```python
from build123d import *

# Parameters (mm, degrees)
SKETCH2_W                      = 60
SKETCH2_H                      = 32
BOSS_EXTRUDE1_DEPTH            = 10
CBORE_FOR_M3_SHCS1_D           = 3.4
CBORE_FOR_M3_SHCS1_CBORE_D     = 6.5
CBORE_FOR_M3_SHCS1_CBORE_DEPTH = 5
SKETCH6_W                      = 17
SKETCH6_H                      = 12
CUT_EXTRUDE2_DEPTH             = 2
CUT_EXTRUDE4_DEPTH             = 5
M5_CLEARANCE_HOLE1_D           = 5.5
SKETCH12_R                     = 2
BOSS_EXTRUDE2_DEPTH            = 2.5
M2X0_4_TAPPED_HOLE1_D          = 1.6
BOSS_EXTRUDE3_DEPTH            = 5
BOSS_EXTRUDE4_DEPTH            = 6.5
FILLET1_R                      = 4
M2X0_4_TAPPED_HOLE2_D          = 1.6
M2X0_4_TAPPED_HOLE2_DEPTH      = 5.2
M2X0_4_TAPPED_HOLE2_TIP        = 0.480688495
CUT_EXTRUDE5_DEPTH             = 3
CHAMFER1_SIZE                  = 1
BOSS_EXTRUDE5_DEPTH            = 10
SKETCH26_R                     = 5.5
CUT_EXTRUDE7_DEPTH             = 14
SKETCH27_R                     = 4
CUT_EXTRUDE8_DEPTH             = 14
FILLET2_R                      = 3
SKETCH28_W                     = 6
SKETCH28_H                     = 6
BOSS_EXTRUDE6_DEPTH            = 10
CUT_EXTRUDE9_DEPTH             = 52.000867623
CUT_EXTRUDE10_REACH            = 76.738
SKETCH30_R                     = 1.6
SKETCH31_R                     = 1.4
CUT_EXTRUDE11_DEPTH            = 5


with BuildPart() as part:
    # Sketch2 → Boss-Extrude1 (new body)
    with BuildSketch(Plane(origin=(0, 0, 0), x_dir=(1, 0, 0), z_dir=(0, 1, 0))):
        Rectangle(SKETCH2_W, SKETCH2_H)
    extrude(amount=BOSS_EXTRUDE1_DEPTH)

    # CBORE for M3 SHCS1 (through all)
    with Locations(Plane(origin=(0, 0, 0), x_dir=(-1, 0, 0), z_dir=(0, -1, 0))):
        with Locations((12.5, 12.5), (12.5, -12.5), (-12.5, -12.5), (-12.5, 12.5)):
            CounterBoreHole(CBORE_FOR_M3_SHCS1_D / 2, CBORE_FOR_M3_SHCS1_CBORE_D / 2, CBORE_FOR_M3_SHCS1_CBORE_DEPTH)

    # Sketch6 → Cut-Extrude2 (cut)
    with BuildSketch(Plane(origin=(0, 0, 0), x_dir=(-1, 0, 0), z_dir=(0, -1, 0))):
        with Locations((0, 10)):
            Rectangle(SKETCH6_W, SKETCH6_H)
    extrude(amount=-CUT_EXTRUDE2_DEPTH, mode=Mode.SUBTRACT)

    # Sketch8 → Cut-Extrude4 (cut)
    with BuildSketch(Plane(origin=(0, 0, -16), x_dir=(-1, 0, 0), z_dir=(0, 0, -1))):
        Polygon((17.265727793, 5), (19.632863896, 0.9), (24.367136104, 0.9), (26.734272207, 5), (24.367136104, 9.1), (19.632863896, 9.1), align=None)
        Polygon((-17.265727793, 5), (-19.632863896, 9.1), (-24.367136104, 9.1), (-26.734272207, 5), (-24.367136104, 0.9), (-19.632863896, 0.9), align=None)
    extrude(amount=-CUT_EXTRUDE4_DEPTH, mode=Mode.SUBTRACT)

    # M5 Clearance Hole1 (through all)
    with Locations(Plane(origin=(0, 0, -11), x_dir=(-1, 0, 0), z_dir=(0, 0, -1))):
        with Locations((22, 5), (-22, 5)):
            Hole(M5_CLEARANCE_HOLE1_D / 2)

    # Sketch12 → Boss-Extrude2 (add)
    with BuildSketch(Plane.XZ):
        with Locations(Location((10.5, -6.5, 0), (0, 0, 180))):
            Circle(SKETCH12_R)
        with Locations((-10.5, -6.5)):
            Circle(SKETCH12_R)
        with Locations(Location((10.5, 6, 0), (0, 0, 90))):
            Circle(SKETCH12_R)
        with Locations(Location((-10.5, 6, 0), (0, 0, 90))):
            Circle(SKETCH12_R)
    extrude(amount=BOSS_EXTRUDE2_DEPTH)

    # M2x0.4 Tapped Hole1 (through all)
    with Locations(Plane(origin=(0, -2.5, 0), x_dir=(-1, 0, 0), z_dir=(0, -1, 0))):
        with Locations((-10.5, -6), (-10.5, 6.5), (10.5, -6), (10.5, 6.5)):
            Hole(M2X0_4_TAPPED_HOLE1_D / 2)

    # Sketch15 → Boss-Extrude3 (add)
    with BuildSketch(Plane(origin=(0, 0, -16), x_dir=(-1, 0, 0), z_dir=(0, 0, -1))):
        Polygon((-13.5, 0), (-13.5, 10), (13.5, 10), (13.5, 0), (8.5, 0), (8.5, 2), (-8.5, 2), (-8.5, 0), align=None)
    extrude(amount=BOSS_EXTRUDE3_DEPTH)

    # Sketch19 → Boss-Extrude4 (add)
    with BuildSketch(Plane(origin=(0, 0, -21), x_dir=(-1, 0, 0), z_dir=(0, 0, -1))):
        Polygon((13.5, 0), (13.5, -6.7), (8.5, -6.7), (8.5, 0), (8.5, 10), (13.5, 10), align=None)
        Polygon((-8.5, 0), (-8.5, 10), (-13.5, 10), (-13.5, 0), (-13.5, -6.7), (-8.5, -6.7), align=None)
    extrude(amount=BOSS_EXTRUDE4_DEPTH)

    # Fillet1
    fillet1_edges = [part.edges().sort_by_distance(p)[0] for p in [
        (-11, 0, -21),
        (11, 0, -21),
    ]]
    fillet(fillet1_edges, radius=FILLET1_R)

    # M2x0.4 Tapped Hole2
    with Locations(Plane(origin=(0, 0, -27.5), x_dir=(-1, 0, 0), z_dir=(0, 0, -1))):
        with Locations((10.75, -4.7), (-10.75, -4.7), (-10.75, 8), (10.75, 8)):
            Hole(M2X0_4_TAPPED_HOLE2_D / 2, depth=M2X0_4_TAPPED_HOLE2_DEPTH)
            with Locations((0, 0, -(M2X0_4_TAPPED_HOLE2_DEPTH + M2X0_4_TAPPED_HOLE2_TIP / 2))):  # 118° drill point
                Cone(0, M2X0_4_TAPPED_HOLE2_D / 2, M2X0_4_TAPPED_HOLE2_TIP, mode=Mode.SUBTRACT)

    # Sketch23 → Cut-Extrude5 (cut)
    with BuildSketch(Plane(origin=(0, 0, -27.5), x_dir=(-1, 0, 0), z_dir=(0, 0, -1))):
        Polygon((8.5, 8), (11.5, 5), (11.5, -1.7), (8.5, -4.7), (-8.5, -4.7), (-11.5, -1.7), (-11.5, 5), (-8.5, 8), align=None)
    extrude(amount=-CUT_EXTRUDE5_DEPTH, mode=Mode.SUBTRACT)

    # Chamfer1
    # the kernel refuses this chamfer: 1 mm, written as the material it adds along each edge
    with BuildSketch(Plane(origin=(10.5, 0, 6), x_dir=(0, 0, 1), z_dir=(1, 0, 0))) as chamfer1_piece_1:
        Polygon((2 + CHAMFER1_SIZE, 0), (2, CHAMFER1_SIZE), (2, 0), align=None)
    revolve(axis=Axis((10.5, 0, 6), (0, -1, 0)))
    with BuildSketch(Plane(origin=(-10.5, 0, -6.5), x_dir=(1, 0, 0), z_dir=(0, 0, -1))) as chamfer1_piece_2_section:
        Polygon((2 + CHAMFER1_SIZE, 0), (2, CHAMFER1_SIZE), (2, 0), align=None)
    chamfer1_piece_2 = revolve(axis=Axis((-10.5, 0, -6.5), (0, -1, 0)), mode=Mode.PRIVATE)
    chamfer1_piece_2 = split(chamfer1_piece_2, bisect_by=Plane(origin=(-8.5, -0.487052851, -6.5), z_dir=(-1, 0, 0)), keep=Keep.TOP, mode=Mode.PRIVATE)
    add(chamfer1_piece_2)
    with BuildSketch(Plane(origin=(-10.5, 0, 6), x_dir=(0, 0, 1), z_dir=(1, 0, 0))) as chamfer1_piece_3:
        Polygon((2 + CHAMFER1_SIZE, 0), (2, CHAMFER1_SIZE), (2, 0), align=None)
    revolve(axis=Axis((-10.5, 0, 6), (0, -1, 0)))
    with BuildSketch(Plane(origin=(10.5, 0, -6.5), x_dir=(-1, 0, 0), z_dir=(0, 0, 1))) as chamfer1_piece_4_section:
        Polygon((2 + CHAMFER1_SIZE, 0), (2, CHAMFER1_SIZE), (2, 0), align=None)
    chamfer1_piece_4 = revolve(axis=Axis((10.5, 0, -6.5), (0, -1, 0)), mode=Mode.PRIVATE)
    chamfer1_piece_4 = split(chamfer1_piece_4, bisect_by=Plane(origin=(8.5, -0.487052851, -6.5), z_dir=(1, 0, 0)), keep=Keep.TOP, mode=Mode.PRIVATE)
    add(chamfer1_piece_4)

    # Sketch25 → Boss-Extrude5 (add)
    with BuildSketch(Plane.XZ):
        Polygon((-30, 0.5), (-30, -6.5), (-30, -13.5), (-41.771263836, -13.5), (-41.771263836, 0.5), align=None)
    extrude(amount=-BOSS_EXTRUDE5_DEPTH)

    # Sketch26 → Cut-Extrude7 (cut)
    with BuildSketch(Plane(origin=(-34.168169597, -5.889190106, 16), x_dir=(-0.888296712324418, -0.45927001956760705, 0), z_dir=(0.45927001956760705, -0.888296712324418, 0))):
        with Locations(Location((-5.5, 22.5, 0), (0, 0, 180))):
            Circle(SKETCH26_R)
    extrude(amount=-CUT_EXTRUDE7_DEPTH, mode=Mode.SUBTRACT)

    # Sketch27 → Cut-Extrude8 (cut, along a direction that is not the sketch's normal)
    with BuildSketch(Plane(origin=(-11.234235046, 21.728686027, 0), x_dir=(0.888296712324418, 0.45927001956760705, 0), z_dir=(0.45927001956760705, -0.888296712324418, 0))):
        with Locations((-27.556201174, -6.5)):
            Circle(SKETCH27_R)
    extrude(amount=-CUT_EXTRUDE8_DEPTH, dir=(0, -1, 0), mode=Mode.SUBTRACT)

    # Fillet2
    fillet2_edges = [part.edges().sort_by_distance(p)[0] for p in [
        (-13.5, 5, -16),
        (13.5, 5, -16),
        (-41.771263836, 5, 0.5),
        (-41.771263836, 5, -13.5),
    ]]
    fillet(fillet2_edges, radius=FILLET2_R)

    # Sketch28 → Boss-Extrude6 (add)
    with BuildSketch(Plane.XZ):
        with Locations((-35.771263836, 3.5)):
            Rectangle(SKETCH28_W, SKETCH28_H)
    extrude(amount=-BOSS_EXTRUDE6_DEPTH)

    # Sketch29 → Cut-Extrude9 (cut, through all)
    with BuildSketch(Plane.XZ):
        Polygon((-30, 0.5), (-31.125452896, -5.882760545), (-33.813152902, -5.408846518), (-32.771263836, 0.5), align=None)
    extrude(amount=-CUT_EXTRUDE9_DEPTH, mode=Mode.SUBTRACT)

    # Sketch30 → Cut-Extrude10 (cut, up to next)
    with BuildSketch(Plane.ZY.offset(38.771263836), mode=Mode.PRIVATE) as cut_extrude10_sk1:
        with Locations((3.5, 5)):
            Circle(SKETCH30_R)
    cut_extrude10_tool1 = extrude(cut_extrude10_sk1.sketch, amount=-CUT_EXTRUDE10_REACH, mode=Mode.PRIVATE) & part.part
    add(cut_extrude10_tool1.solids().sort_by_distance((-38.771264, 5, 3.5))[0], mode=Mode.SUBTRACT)

    # Sketch31 → Cut-Extrude11 (cut)
    with BuildSketch(Plane.ZY.offset(30)):
        with Locations((3.5, 5)):
            Circle(SKETCH31_R)
    extrude(amount=-CUT_EXTRUDE11_DEPTH, mode=Mode.SUBTRACT)


solid = part.part
```
Model file for the job. Use its own axes, mm. A direction names the side the tool comes from. Round coordinates to 2 decimals unless told otherwise and drop trailing zeros. Order: outer loops, then holes, each group sorted by start corner. A loop starts at its lowest first (then second) coordinate and runs counter-clockwise, first axis right, second up. Notation, with made-up numbers: (34, 76.5) -> (77, 76.5) arc R11 ccw to (77, 89.5) -> close; hole circle Ø6 at (-38.75, 15.25). An arc over 180 degrees is marked (long way). Use one line per item in the form item = value.
Item 1: Flat gauge pins, fed straight in: pin 1 Ø8 at (y, z) = (6, -21.5) entering from +X; pin 2 Ø8 at (x, y) = (21, 3) entering from -Z; pin 3 Ø5 at (x, y) = (14, 6) entering from -Z; pin 4 Ø1.5 at (x, y) = (22.5, 5) entering from +Z. Where does each tip first touch, or does it go through?
Returned:
pin_1 = 13.9
pin_2 = -16
pin_3 = -27.5
pin_4 = through
Item 2: Tool access for faces 1 (the face through (-38.771, 4, 2)), 2 (the face through (9.6, -2.5, -6.1)), 3 (the face through (-10.105, 2.465, 10.303)), 4 (the face through (-22, 0.9, -14)), 5 (the face through (-32.771, 4, 2)): list every direction of +Z, -Z, +X, -X, +Y, -Y with a clear straight run to the whole face (end or side of a thin tool).
Returned:
face_1 = +Z, -X, +Y, -Y
face_2 = +Z, +X, -X, -Y
face_3 = -Y
face_4 = -Z
face_5 = +Z, +Y, -Y
Item 3: Cut at A-A, the plane x = 22. Write the cut outline in (y, z), and give its area (4 significant figures).
Returned:
outline = (0, -16) -> (0.9, -16) -> (0.9, -11) -> (2.25, -11) -> (2.25, 16) -> (0, 16) -> close; (7.75, -11) -> (9.1, -11) -> (9.1, -16) -> (10, -16) -> (10, 16) -> (7.75, 16) -> close
area = 130.5 mm^2
Item 4: Pull direction Z, two halves, no side cores. Call faces 6 (the face through (-9.253, 2.465, -12.643)), 7 (the face through (-22, 9.1, -14)), 8 (the face through (-10.611, 8.006, -21.903)): released by +Z, released by -Z, zero draft, split by the parting line, or undercut.
Returned:
face_6 = undercut
face_7 = zero draft
face_8 = released by -Z
Item 5: Cut at C-C, the plane x = 2. Write the cut outline in (y, z), and give its area (3 significant figures).
Returned:
outline = (0, -4) -> (2, -4) -> (2, -21) -> (10, -21) -> (10, 16) -> (0, 16) -> close
area = 336 mm^2
Item 6: Cut at B-B, the plane z = 11.5. Write the cut outline in (x, y), and give its area (3 significant figures).
Returned:
outline = (-30, 0) -> (-15.59, 0) -> (-15.59, 5) -> (-13.87, 5) -> (-13.87, 10) -> (-30, 10) -> close; (-11.13, 5) -> (-9.41, 5) -> (-9.41, 0) -> (9.41, 0) -> (9.41, 5) -> (11.13, 5) -> (11.13, 10) -> (-11.13, 10) -> close; (13.87, 5) -> (15.59, 5) -> (15.59, 0) -> (30, 0) -> (30, 10) -> (13.87, 10) -> close; hole circle Ø5.5 at (-22, 5); hole circle Ø5.5 at (22, 5)
area = 463 mm^2
Item 7: Drill centre lines: line 1 (Z direction, x = -12.5, y = 3.3); line 2 (Z direction, x = 10.5, y = 5.75); line 3 (X direction, y = -1.75, z = -22). Where is each one in solid material? Low to high.
Returned:
line_1 = -27.5 to -15.75, -9.25 to 9.25, 15.75 to 16
line_2 = -24.5 to -7.3, -5.7 to 5.2, 6.8 to 16
line_3 = -13.5 to -8.5, 8.5 to 13.5
